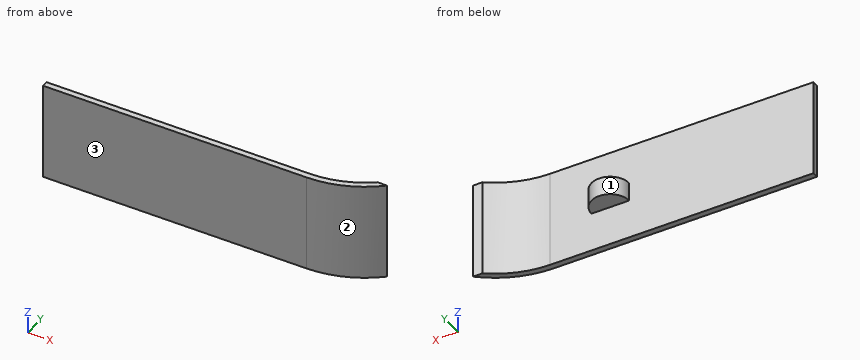
```python
from build123d import *

# Parameters (mm, degrees)
F0_W          = 70
F0_H          = 1.6
F1_DEPTH      = 13
F1_DEPTH_BACK = 13
F2_W          = 5
F2_H          = 5
F3_ANGLE      = 180


with BuildPart() as f1:
    # F0 (on Top) → F1 (new body, two sides)
    with BuildSketch(Plane.XY) as f1_sk:
        with Locations((-35, 0.8)):
            Rectangle(F0_W, F0_H)
        with BuildLine():
            Line((0, 1.6), (0, 0))
            ThreePointArc((0, 0), (9.369098, 1.704619), (17.537389, 6.6))
            Line((17.537389, 6.6), (15, 6.6))
            ThreePointArc((15, 6.6), (7.905694, 2.882918), (0, 1.6))
        make_face()
    extrude(amount=F1_DEPTH)
    extrude(f1_sk.sketch, amount=-F1_DEPTH_BACK)

    # F2 (on face) → F3 (revolve)
    with BuildSketch(Plane(origin=(0, 1.6, 0), x_dir=(-1, 0, 0), z_dir=(0, 1, 0))):
        with Locations((18.5, 0)):
            Rectangle(F2_W, F2_H)
    revolve(axis=Axis((-16, 1.6, 0), (0, 0, -1)), revolution_arc=F3_ANGLE)


solid = f1.part
```
The model under review builds one solid part; all positions refer to its coordinate system, in mm. Face numbers are marked on the shaded views. Coordinates: 2 decimals unless noted, no trailing zeros. Write each loop counter-clockwise with the first axis right and the second up, starting at its lowest first coordinate (ties: lowest second). Pieces come first, ordered by that corner, then holes. Notation, with made-up numbers: (40, -18.5) -> (93, -18.5) arc R20 ccw to (93, 14.5) -> close; hole circle Ø3 at (-2.75, -33). An arc over 180 degrees is marked (long way). One line per item, written item: value. Start each with the question number.
Q1. Add section D-D, the plane z = 3.25. Give the boundary of the cut face in (x, y).
Q2. To check wall thickness, follow probe 1 along Y at (x, z) = (-41, 6.5); probe 2 along X at (y, z) = (4.75, 1); probe 3 along Z at (x, y) = (-16.5, 3.5). State the ranges of each line that lie inside material, in increasing order.
Q3. Add section B-B, the plane z = -0.25. Give the boundary of the cut face in (x, y), then the cut area to 3 significant figures.
Q4. Add section C-C, the plane y = 4.5. Give the boundary of the cut face in (x, z).
Q5. Add section A-A, the plane x = -16. Give the boundary of the cut face in (y, z).
Q6. The part is to be moulded in two halves that separate along X. For the marked faces 1, 2 and 3, say which applies: +X half, -X half, draft (parallel to the pull), parting line (faces both ways), or undercut.
Q7. Clearance check with flat-ended pins moving along their axes: P1, Ø2.5, axis at x = -15.5, y = 5, coming from the +Z side; P2, Ø2, axis at x = -15.5, z = -5, coming from the +Y side; P3, Ø2.5, axis at x = -15, y = 3.5, coming from the -Z side. State where each tip first meets the part, or that it passes through.
Response:
1. outline: (-70, 0) -> (0, 0) arc R26.6 ccw to (17.54, 6.6) -> (15, 6.6) arc R25 cw to (0, 1.6) -> (-70, 1.6) -> close
2. probe 1: 0 to 1.6
2. probe 2: -19.88 to -12.12, 12.15 to 15.17
2. probe 3: -2.5 to 2.5
3. outline: (-70, 0) -> (0, 0) arc R26.6 ccw to (17.54, 6.6) -> (15, 6.6) arc R25 cw to (0, 1.6) -> (-11, 1.6) arc R5 ccw to (-21, 1.6) -> (-70, 1.6) -> close
3. area: 179 mm²
4. outline: (-20.07, -2.5) -> (-11.93, -2.5) -> (-11.93, 2.5) -> (-20.07, 2.5) -> close; (11.69, -13) -> (14.8, -13) -> (14.8, 13) -> (11.69, 13) -> close
5. outline: (0, -13) -> (1.6, -13) -> (1.6, -2.5) -> (6.6, -2.5) -> (6.6, 2.5) -> (1.6, 2.5) -> (1.6, 13) -> (0, 13) -> close
6. face 1: undercut
6. face 2: +X half
6. face 3: draft
7. P1: z = 2.5
7. P2: y = 1.6
7. P3: z = -2.5
